Here's how the part is built. I have some questions about the finished solid (model axes, mm). A direction names the side the tool comes from. Coordinates: 2 decimals unless noted, no trailing zeros. Write each loop counter-clockwise with the first axis right and the second up, starting at its lowest first coordinate (ties: lowest second). Pieces come first, ordered by that corner, then holes. Notation, with made-up numbers: (89.25, -39.5) -> (142.25, -39.5) arc R36 ccw to (142.25, -2.5) -> close; hole circle Ø4 at (26.5, 73). An arc over 180 degrees is marked (long way). Use a Markdown table: item, result. Add a question column.
Item 1: Will these pins go through, and if not, where does the flat tip stop? pin 1 Ø1.5 at (y, z) = (-3.5, 11.5) entering from +X; pin 2 Ø2 at (y, z) = (-3, 14) entering from +X; pin 3 Ø1.5 at (y, z) = (-1.5, 13) entering from -X.
Item 2: If we mould it in two halves opening along Z, with no side actions, what happens to faces 1 (the flat face through (0, -4, 12.8)), 2 (the flat face through (0, -4, 15.272)), 3 (the cylindrical face through (-1.341, 3.233, 18.145)), 4 (the flat face through (-2, 2, 6.5))? For each: pulls with the +Z half, pulls with the -Z half, needs draft (parallel to the pull), parting line crosses it, or undercut.
Item 3: Imagine slicing it at D-D, the plane z = 13.25. Write out the boundary of the cut face in (x, y).
Item 4: If I drill on line 1 along Z through (x, y) = (2.5, -4); line 2 along Z through (x, y) = (-1.75, -2.5); line 3 along X through (y, z) = (0.25, 7.5), over which ranges is the centre line in solid material (lowest first)? Write a range as from..to.
Item 5: On a 3-axis mill with a long thin cutter (end or side, diameter ignored), from which of +Z, -Z, +X, -X, +Y, -Y can I reach the whole of each face in a straight line? I mean faces 5 (the flat face through (0, 0, 21.1)), 6 (the flat face through (2, -2, 4.517)), 7 (the cylindrical face through (0, -3, 2)). Say none if no direction works.
Item 6: Imagine slicing it at C-C, the plane z = 7. Write out the boundary of the cut face in (x, y), and give its area (3 significant figures).
Item 7: Imagine slicing it at A-A, the plane y = 0. Write out the boundary of the cut face in (x, z).
Autodesk Inventor part; units mm, degrees
ref_plane "YZ Plane" through (0, 0, 0) normal (1, 0, 0) x (0, 1, 0)
ref_plane "XZ Plane" through (0, 0, 0) normal (0, 1, 0) x (-1, 0, 0)
ref_plane "XY Plane" through (0, 0, 0) normal (0, 0, 1) x (1, 0, 0)
sketch "Sketch1" plane through (0, 0, 0) normal (1, 0, 0) x (0, 1, 0)
  line L0 (0, 21.1) -> (3.5, 21.1)
  line L1 (3.5, 21.1) -> (3.5, 15.2717)
  line L2 (3.5, 15.2717) -> (4.75, 15.2717)
  line L3 (4.75, 15.2717) -> (4.75, 12.8)
  line L4 (4.75, 12.8) -> (3.5, 12.8)
  line L5 (3.5, 12.8) -> (3.5, 6.5)
  line L6 (3.5, 6.5) -> (2.5, 6.5)
  line L7 (2.5, 6.5) -> (2.5, 4.517)
  line L8 (2.5, 4.517) -> (3, 4.517)
  line L9 (3, 4.517) -> (3, 0)
  line L10 (3, 0) -> (0, 0)
  line L11 (0, 21.1) -> (0, 0)
  dimension "d0" = 21.1
  dimension "d1" = 3
  dimension "d2" = 3.5
  dimension "d3" = 2.5
  dimension "d4" = 6.5
  dimension "d5" = 4.517
  dimension "d6" = 6.3
  dimension "d7" = 2.4717
  dimension "d8" = 4.75
revolve "Revolution1" add sketch "Sketch1" angle 360 about axis through (0, 0, 21.1) along (0, 0, -1)
properties part number "Button" material "Nylon 6/6"
Ans:
| question | item | result |
|---|---|---|
| 1 | pin 1 | stops at x = 2.17 |
| 1 | pin 2 | stops at x = 4.31 |
| 1 | pin 3 | stops at x = -4.69 |
| 2 | face 1 | pulls with the -Z half |
| 2 | face 2 | pulls with the +Z half |
| 2 | face 3 | needs draft |
| 2 | face 4 | undercut |
| 3 | outline | circle Ø9.5 at (0, 0) |
| 4 | line 1 | z = 12.8..15.27 |
| 4 | line 2 | z = 6.5..21.1 |
| 4 | line 3 | x = -3.49..3.49 |
| 5 | face 5 | +Z, +X, -X, +Y, -Y |
| 5 | face 6 | none |
| 5 | face 7 | -Z |
| 6 | outline | circle Ø7 at (0, 0) |
| 6 | area | 38.5 mm^2 |
| 7 | outline | (-4.75, 12.8) -> (-3.5, 12.8) -> (-3.5, 6.5) -> (-2.5, 6.5) -> (-2.5, 4.52) -> (-3, 4.52) -> (-3, 0) -> (3, 0) -> (3, 4.52) -> (2.5, 4.52) -> (2.5, 6.5) -> (3.5, 6.5) -> (3.5, 12.8) -> (4.75, 12.8) -> (4.75, 15.27) -> (3.5, 15.27) -> (3.5, 21.1) -> (-3.5, 21.1) -> (-3.5, 15.27) -> (-4.75, 15.27) -> close |
